Read the model definition and answer for the solid it produces. Units are mm, in the model's axes. A direction names the side the tool comes from. Give positions to 0.01 mm unless a question says otherwise; leave off trailing zeros. Loops run counter-clockwise (first coordinate to the right, second up) from the corner with the lowest first, then second, coordinate; pieces in that order, holes last. Notation, with made-up numbers: (-4, 51) -> (15, 51) arc R21 cw to (15, 76) -> close; hole circle Ø4 at (3.5, -28.75). An arc over 180 degrees is marked (long way). One line per item, written item: value. Start each with the question number.
from build123d import *

# Parameters (mm, degrees)
SKETCH1_2_R                 = 2.65
EXTRUDE_1_DEPTH             = 200
HOLE_WIZARD_M5_1_AT_2_COUNT = 2
HOLE_WIZARD_M5_1_AT_2_PITCH = 30


# Read off the part's stored shape, not the designer's step: 30 x 60G x R1.5<1>
with BuildPart() as part:
    # Sketch1<2> → 凸台-拉伸1 (new body)
    with BuildSketch(Plane(origin=(1.902137601, -4.901792835, 0), x_dir=(1, 0, 0), z_dir=(0, 0, 1))):
        with BuildLine():
            Line((-3.25, 30), (-3.25, 29))
            Line((-3.25, 29), (-4.25, 29))
            Line((-4.25, 29), (-4.25, 21.277812156))
            ThreePointArc((-4.25, 21.277812156), (0, 20.5), (4.25, 21.277812156))
            Line((4.25, 21.277812156), (4.25, 29))
            Line((4.25, 29), (3.25, 29))
            Line((3.25, 29), (3.25, 30))
            Line((3.25, 30), (13.5, 30))
            ThreePointArc((13.5, 30), (14.560660172, 29.560660172), (15, 28.5))
            Line((15, 28.5), (15, 18.25))
            Line((15, 18.25), (14, 18.25))
            Line((14, 18.25), (14, 19.25))
            Line((14, 19.25), (6.277812156, 19.25))
            ThreePointArc((6.277812156, 19.25), (5.5, 15), (6.277812156, 10.75))
            Line((6.277812156, 10.75), (14, 10.75))
            Line((14, 10.75), (14, 11.75))
            Line((14, 11.75), (15, 11.75))
            Line((15, 11.75), (15, -11.75))
            Line((15, -11.75), (14, -11.75))
            Line((14, -11.75), (14, -10.75))
            Line((14, -10.75), (6.277812156, -10.75))
            ThreePointArc((6.277812156, -10.75), (5.5, -15), (6.277812156, -19.25))
            Line((6.277812156, -19.25), (14, -19.25))
            Line((14, -19.25), (14, -18.25))
            Line((14, -18.25), (15, -18.25))
            Line((15, -18.25), (15, -28.5))
            ThreePointArc((15, -28.5), (14.560660172, -29.560660172), (13.5, -30))
            Line((13.5, -30), (3.25, -30))
            Line((3.25, -30), (3.25, -29))
            Line((3.25, -29), (4.25, -29))
            Line((4.25, -29), (4.25, -21.277812156))
            ThreePointArc((4.25, -21.277812156), (0, -20.5), (-4.25, -21.277812156))
            Line((-4.25, -21.277812156), (-4.25, -29))
            Line((-4.25, -29), (-3.25, -29))
            Line((-3.25, -29), (-3.25, -30))
            Line((-3.25, -30), (-13.5, -30))
            ThreePointArc((-13.5, -30), (-14.560660172, -29.560660172), (-15, -28.5))
            Line((-15, -28.5), (-15, -18.25))
            Line((-15, -18.25), (-14, -18.25))
            Line((-14, -18.25), (-14, -19.25))
            Line((-14, -19.25), (-6.277812156, -19.25))
            ThreePointArc((-6.277812156, -19.25), (-5.5, -15), (-6.277812156, -10.75))
            Line((-6.277812156, -10.75), (-14, -10.75))
            Line((-14, -10.75), (-14, -11.75))
            Line((-14, -11.75), (-15, -11.75))
            Line((-15, -11.75), (-15, 11.75))
            Line((-15, 11.75), (-14, 11.75))
            Line((-14, 11.75), (-14, 10.75))
            Line((-14, 10.75), (-6.277812156, 10.75))
            ThreePointArc((-6.277812156, 10.75), (-5.5, 15), (-6.277812156, 19.25))
            Line((-6.277812156, 19.25), (-14, 19.25))
            Line((-14, 19.25), (-14, 18.25))
            Line((-14, 18.25), (-15, 18.25))
            Line((-15, 18.25), (-15, 28.5))
            ThreePointArc((-15, 28.5), (-14.560660172, 29.560660172), (-13.5, 30))
            Line((-13.5, 30), (-3.25, 30))
        make_face()
        with Locations((-11, 26)):
            Circle(SKETCH1_2_R, mode=Mode.SUBTRACT)
        with Locations(Location((11, 26, 0), (0, 0, 180))):
            Circle(SKETCH1_2_R, mode=Mode.SUBTRACT)
        with Locations((11, -26)):
            Circle(SKETCH1_2_R, mode=Mode.SUBTRACT)
        with Locations(Location((-11, -26, 0), (0, 0, 180))):
            Circle(SKETCH1_2_R, mode=Mode.SUBTRACT)
        with BuildLine():
            Line((-12.5, 7.5), (-4, 7.5))
            Line((-4, 7.5), (-1.665625283, 13.135679101))
            ThreePointArc((-1.665625283, 13.135679101), (0, 17.5), (1.665625283, 13.135679101))
            Line((1.665625283, 13.135679101), (4, 7.5))
            Line((4, 7.5), (12.5, 7.5))
            Line((12.5, 7.5), (12.5, -7.5))
            Line((12.5, -7.5), (4, -7.5))
            Line((4, -7.5), (1.665625283, -13.135679101))
            ThreePointArc((1.665625283, -13.135679101), (0, -17.5), (-1.665625283, -13.135679101))
            Line((-1.665625283, -13.135679101), (-4, -7.5))
            Line((-4, -7.5), (-12.5, -7.5))
            Line((-12.5, -7.5), (-12.5, 7.5))
        make_face(mode=Mode.SUBTRACT)
    extrude(amount=EXTRUDE_1_DEPTH)

    # 草图4 → M5 螺纹孔1 (revolve, cut)
    with BuildSketch(Plane(origin=(-13.097862399, -4.901792835, 45), x_dir=(0, 0, 1), z_dir=(0, 1, 0))):
        Polygon((0, 0), (0, 2.5), (2.1, 2.5), (2.1, 0.425), (2.525, 0), align=None)
    hole_wizard_m5_1 = revolve(axis=Axis((-19.447862399, -4.901792835, 45), (1, 0, 0)), mode=Mode.SUBTRACT)

    # M5 螺纹孔1 at 2: M5 螺纹孔1 ×2
    with Locations(*[(0, 0, -i * HOLE_WIZARD_M5_1_AT_2_PITCH) for i in range(1, HOLE_WIZARD_M5_1_AT_2_COUNT)]):
        add(hole_wizard_m5_1, mode=Mode.SUBTRACT)


solid = part.part
Item 1: Section B-B, the plane x = -8.5 is taken. Determine the outline of the cut face in (y, z), plus the area to 3 significant figures.
Item 2: Section A-A, the plane y = 0.5 is taken. Determine the outline of the cut face in (x, z), plus the area to 3 significant figures.
Item 3: For faces 1 (the cylindrical face through (1.96, -25.4, 98.6)), 2 (the flat face through (16.902, -5, 99)), determine the directions among +Z, -Z, +X, -X, +Y, -Y from which every point of the face is accessible in a straight line to the end or side of a thin tool.
Item 4: Flat-ended cylindrical pins translate along their axes: pin 1 (1.1 mm diameter, centred on x = -12.5, z = 148, fed in from +Y); pin 2 (1.5 mm diameter, centred on y = -21, z = 23.5, fed in from +X); pin 3 (0.5 mm diameter, centred on y = 24.5, z = 142.5, fed in from +X). Find the tip coordinate at first contact, or state that the pin passes through.
Item 5: Section D-D, the plane z = 45 is taken. State how many separate pieces and enclosed holes the cut face has, plus the area to 3 significant figures.
Item 6: Section C-C, the plane x = 12 is taken. Determine the outline of the cut face in (y, z), plus the area to 3 significant figures.
Item 7: Consider L1, parallel to Y at x = 10, z = 171; L2, parallel to X at y = -4, z = 140.5; L3, parallel to X at y = 18, z = 127.5. Determine where each line is inside the solid, lowest interval first. Write a range as [from, to].
Item 8: Determine the mould class of faces 3 (the flat face through (5, 9, 0)), 4 (the cylindrical face through (1.8, 15.6, 98.6)), 5 (the cylindrical face through (-11.65, -4.99, 12.9)), 6 (the flat face through (5, 9, 200)) for opening direction Z: pulls with the +Z half, pulls with the -Z half, needs draft (parallel to the pull), parting line crosses it, or undercut.
Computed values:
1. outline: (-34.9, 0) -> (-33.48, 0) -> (-33.48, 200) -> (-34.9, 200) -> close; (-28.32, 0) -> (-24.15, 0) -> (-24.15, 200) -> (-28.32, 200) -> close; (-15.65, 0) -> (-12.4, 0) -> (-12.4, 200) -> (-15.65, 200) -> close; (2.6, 0) -> (5.85, 0) -> (5.85, 200) -> (2.6, 200) -> close; (14.35, 0) -> (18.52, 0) -> (18.52, 200) -> (14.35, 200) -> close; (23.68, 0) -> (25.1, 0) -> (25.1, 200) -> (23.68, 200) -> close
1. area: 3,530 mm²
2. outline: (-13.1, 0) -> (-10.6, 0) -> (-10.6, 200) -> (-13.1, 200) -> close; (14.4, 0) -> (16.9, 0) -> (16.9, 200) -> (14.4, 200) -> close
2. area: 1,000 mm²
3. face 1: +Z, -Z
3. face 2: +Z, -Z, +X, +Y, -Y
4. pin 1: y = 25.06
4. pin 2: x = 7.55
4. pin 3: x = 16.75
5. separate pieces: 1
5. enclosed holes: 4
5. area: 764 mm²
6. outline: (-34.9, 0) -> (-33.39, 0) -> (-33.39, 200) -> (-34.9, 200) -> close; (-28.41, 0) -> (-24.15, 0) -> (-24.15, 200) -> (-28.41, 200) -> close; (-15.65, 0) -> (-12.4, 0) -> (-12.4, 200) -> (-15.65, 200) -> close; (2.6, 0) -> (5.85, 0) -> (5.85, 200) -> (2.6, 200) -> close; (14.35, 0) -> (18.61, 0) -> (18.61, 200) -> (14.35, 200) -> close; (23.59, 0) -> (25.1, 0) -> (25.1, 200) -> (23.59, 200) -> close
6. area: 3,610 mm²
7. L1: [-34.9, -24.15], [-15.65, -12.4], [2.6, 5.85], [14.35, 25.1]
7. L2: [-13.1, -10.6], [14.4, 16.9]
7. L3: [-13.1, -2.35], [6.15, 16.9]
8. face 3: pulls with the -Z half
8. face 4: needs draft
8. face 5: undercut
8. face 6: pulls with the +Z half
